Here's how the part is built. I have some questions about the finished solid (model axes, mm). A direction names the side the tool comes from. Round coordinates to 2 decimals unless told otherwise and drop trailing zeros. Write each loop counter-clockwise with the first axis right and the second up, starting at its lowest first coordinate (ties: lowest second). Pieces come first, ordered by that corner, then holes. Notation, with made-up numbers: (-5.75, 44) - (36.25, 44) arc R25 cw to (36.25, 62) - close; hole circle Ø9 at (32, 18.25). An arc over 180 degrees is marked (long way). Write item = value, one per line. Start each with the question number.
Item 1: Thinking about a two-plate mould opening in X: for faces 3 (the face through (-10.4, 0.1, 1.5)), 4 (the face through (-32, 0, 2)), 5 (the face through (32, 0, 2)), 6 (the face through (0, 0, 0)), which applies, pulls with the +X half, pulls with the -X half, needs draft (parallel to the pull), parting line crosses it, or undercut?
Item 2: If we section it at C-C (z = 1): Please give me the cut outline in (x, y), and give its area (3 significant figures).
Item 3: If I drill on line 1 along X through (y, z) = (0, 3.7); line 2 along Y through (x, z) = (7.5, 1.9); line 3 along Y through (x, z) = (22.5, 3.55), over which ranges is the centre line in solid material (lowest first)? Write a range as [from, to].
Item 4: If we section it at D-D (y = 0): Give the number of separate pieces and of enclosed holes in the cut face, and give its area (3 significant figures).
Item 5: For P1, Ø4.5, axis at x = -8.5, y = -0.5, coming from the -Z side; P2, Ø3, axis at x = 6.5, y = -1, coming from the -Z side, each with a flat end and sliding along its axis, tell me the tip position at first contact or that it passes through.
Item 6: If we section it at B-B (x = -22.5): Please give me the cut outline in (y, z), and give its area (3 significant figures).
Item 7: Which directions (+Z, -Z, +X, -X, +Y, -Y) give clear straight access to the entire face, cutting with the end or side of a thin tool? Please do faces 1 (the face through (-8.85, -1.03, 3.49)), 2 (the face through (19.5, 0.1, 1.5)).
Item 8: If we section it at A-A (y = 5): Please give me the cut outline in (x, z), and give its area (3 significant figures).
```python
from build123d import *

# Parameters (mm, degrees)
COUPON_BAR_64X14X4_PROFILE_W                   = 64
COUPON_BAR_64X14X4_PROFILE_H                   = 14
COUPON_BAR_64X14X4_DEPTH                       = 4
PRESS_SOCKETS_5P70_5P80_5P90_6P00_DE_2_R       = 2.85
PRESS_SOCKETS_5P70_5P80_5P90_6P00_DE_2_R_2     = 2.9
PRESS_SOCKETS_5P70_5P80_5P90_6P00_DE_2_R_3     = 2.95
PRESS_SOCKETS_5P70_5P80_5P90_6P00_DE_2_R_4     = 3
PRESS_SOCKETS_5P70_5P80_5P90_6P00_DEPTH3_DEPTH = 3
M3_CENTRE_SCREW_CLEARANCE_START                = -50
M3_CENTRE_SCREW_CLEARANCE_PROFILE_R            = 1.7
M3_CENTRE_SCREW_CLEARANCE_DEPTH                = 84
ORIENTATION_MARK_AT_SMALLEST_SOCKET_START      = -50
ORIENTATION_MARK_AT_SMALLEST_SOCKET_PROF_R     = 0.75
ORIENTATION_MARK_AT_SMALLEST_SOCKET_DEPTH      = 84


with BuildPart() as part:
    # Coupon_bar_64x14x4_profile → Coupon_bar_64x14x4 (new body)
    with BuildSketch(Plane.XY):
        Rectangle(COUPON_BAR_64X14X4_PROFILE_W, COUPON_BAR_64X14X4_PROFILE_H)
    extrude(amount=COUPON_BAR_64X14X4_DEPTH)

    # Press_sockets_5p70_5p80_5p90_6p00_de 2 → Press_sockets_5p70_5p80_5p90_6p00_depth3 (cut)
    with BuildSketch(Plane.XY):
        with Locations((-22.5, 0)):
            Circle(PRESS_SOCKETS_5P70_5P80_5P90_6P00_DE_2_R)
        with Locations((-7.5, 0)):
            Circle(PRESS_SOCKETS_5P70_5P80_5P90_6P00_DE_2_R_2)
        with Locations((7.5, 0)):
            Circle(PRESS_SOCKETS_5P70_5P80_5P90_6P00_DE_2_R_3)
        with Locations((22.5, 0)):
            Circle(PRESS_SOCKETS_5P70_5P80_5P90_6P00_DE_2_R_4)
    extrude(amount=PRESS_SOCKETS_5P70_5P80_5P90_6P00_DEPTH3_DEPTH, mode=Mode.SUBTRACT)

    # M3_centre_screw_clearance_profile → M3_centre_screw_clearance (cut, through all)
    with BuildSketch(Plane.XY.offset(M3_CENTRE_SCREW_CLEARANCE_START)):
        with Locations((-22.5, 0)):
            Circle(M3_CENTRE_SCREW_CLEARANCE_PROFILE_R)
        with Locations((-7.5, 0)):
            Circle(M3_CENTRE_SCREW_CLEARANCE_PROFILE_R)
        with Locations((7.5, 0)):
            Circle(M3_CENTRE_SCREW_CLEARANCE_PROFILE_R)
        with Locations((22.5, 0)):
            Circle(M3_CENTRE_SCREW_CLEARANCE_PROFILE_R)
    extrude(amount=M3_CENTRE_SCREW_CLEARANCE_DEPTH, mode=Mode.SUBTRACT)

    # Orientation_mark_at_smallest_socket_profile → Orientation_mark_at_smallest_socket (cut, through all)
    with BuildSketch(Plane.XY.offset(ORIENTATION_MARK_AT_SMALLEST_SOCKET_START)):
        with Locations(Location((-30, 5, 0), (0, 0, 180))):
            Circle(ORIENTATION_MARK_AT_SMALLEST_SOCKET_PROF_R)
    extrude(amount=ORIENTATION_MARK_AT_SMALLEST_SOCKET_DEPTH, mode=Mode.SUBTRACT)


solid = part.part
```
Reply:
q1.face_3 = undercut
q1.face_4 = pulls with the -X half
q1.face_5 = pulls with the +X half
q1.face_6 = needs draft
q2.outline = (-32, -7) - (32, -7) - (32, 7) - (-32, 7) - close; hole circle Ø1.5 at (-30, 5); hole circle Ø5.7 at (-22.5, 0); hole circle Ø5.8 at (-7.5, 0); hole circle Ø5.9 at (7.5, 0); hole circle Ø6 at (22.5, 0)
q2.area = 787 mm2
q3.line_1 = [-32, -24.2], [-20.8, -9.2], [-5.8, 5.8], [9.2, 20.8], [24.2, 32]
q3.line_2 = [-7, -2.95], [2.95, 7]
q3.line_3 = [-7, -1.7], [1.7, 7]
q4.separate_pieces = 5
q4.enclosed_holes = 0
q4.area = 172 mm2
q5.P1 = 0
q5.P2 = 3
q6.outline = (-7, 0) - (-2.85, 0) - (-2.85, 3) - (-1.7, 3) - (-1.7, 4) - (-7, 4) - close; (1.7, 3) - (2.85, 3) - (2.85, 0) - (7, 0) - (7, 4) - (1.7, 4) - close
q6.area = 35.5 mm2
q7.face_1 = +Z, -Z
q7.face_2 = -Z
q8.outline = (-32, 0) - (-30.75, 0) - (-30.75, 4) - (-32, 4) - close; (-29.25, 0) - (32, 0) - (32, 4) - (-29.25, 4) - close
q8.area = 250 mm2
